from build123d import *

# Parameters (mm, degrees)
F0_W      = 16.51
F0_H      = 21.59
F1_DEPTH  = 3.048
F2_W      = 1.7145
F2_H      = 12.7
F3_DEPTH  = 25.4
F4_W      = 1.5875
F4_H      = 12.7
F5_DEPTH  = 25.4
F7_DEPTH  = 25.4
F8_R      = 1.52399
F9_R      = 1.524
F10_DEPTH = 2.286
F11_R     = 1.524
F12_DEPTH = 2.286
F13_R     = 0.635
F14_R     = 0.635


# Not quite as in the source:
# - a fillet or chamfer is up to 0.001 mm smaller than in the source, because OpenCascade refuses the exact size


with BuildPart() as f1:
    # F0 (on Top) → F1 (new body)
    with BuildSketch(Plane.XY):
        with Locations((8.255, 10.795)):
            Rectangle(F0_W, F0_H)
    extrude(amount=F1_DEPTH)

    # F2 (on face) → F3 (cut)
    with BuildSketch(Plane.XY.offset(3.048)):
        with Locations((4.03225, 15.24)):
            Rectangle(F2_W, F2_H)
    extrude(amount=-F3_DEPTH, mode=Mode.SUBTRACT)

    # F4 (on face) → F5 (cut)
    with BuildSketch(Plane.XY.offset(3.048)):
        with Locations((12.54125, 15.24)):
            Rectangle(F4_W, F4_H)
    extrude(amount=-F5_DEPTH, mode=Mode.SUBTRACT)

    # F6 (on face) → F7 (cut)
    with BuildSketch(Plane(origin=(0, 0, 0), x_dir=(0, -1, 0), z_dir=(-1, 0, 0))):
        Polygon((0, 0), (0, 3.048), (-3.175, 0), align=None)
    extrude(amount=-F7_DEPTH, mode=Mode.SUBTRACT)

    # F8 (radius 1.524 in the source; OpenCascade refuses exactly that, so slightly less here)
    f8_edges = [f1.edges().sort_by_distance(p)[0] for p in [
        (1.5875, 21.59, 3.048),
        (1.5875, 21.59, 0),
        (8.3185, 21.59, 3.048),
        (8.3185, 21.59, 0),
        (14.9225, 21.59, 3.048),
        (14.9225, 21.59, 0),
    ]]
    fillet(f8_edges, radius=F8_R)

    # F9 (on face) → F10 (join)
    with BuildSketch(Plane(origin=(0, 0, 0), x_dir=(0, -1, 0), z_dir=(-1, 0, 0))):
        with Locations((-20.066, 1.524)):
            Circle(F9_R)
    extrude(amount=F10_DEPTH)

    # F11 (on face) → F12 (join)
    with BuildSketch(Plane.YZ.offset(16.51)):
        with Locations((20.066, 1.524)):
            Circle(F11_R)
    extrude(amount=F12_DEPTH)

    # F13
    f13_edges = [f1.edges().sort_by_distance(p)[0] for p in [
        (18.796, 18.542, 1.524),
        (-2.286, 21.59, 1.524),
    ]]
    fillet(f13_edges, radius=F13_R)

    # F14
    f14_edges = [f1.edges().sort_by_distance(p)[0] for p in [
        (11.7475, 8.89, 1.524),
        (13.335, 8.89, 1.524),
        (3.175, 8.89, 1.524),
        (4.8895, 8.89, 1.524),
    ]]
    fillet(f14_edges, radius=F14_R)


solid = f1.part
For this review, take the finished solid that the model builds, in its own axes (mm). A direction names the side the tool comes from. Give positions to 0.01 mm unless a question says otherwise; leave off trailing zeros. Loops run counter-clockwise (first coordinate to the right, second up) from the corner with the lowest first, then second, coordinate; pieces in that order, holes last.
Item 1: Draft analysis for pull direction X (two halves, no side actions). For faces 1 (the flat face through (0, 10, 2)), 2 (the flat face through (4.89, 15, 2)), 3 (the flat face through (8, 12, 0)), state which applies: +X half, -X half, draft (parallel to the pull), parting line (faces both ways), or undercut.
Item 2: Tool access review of faces 4 (the cylindrical face through (17.324, 18.543, 1.591)), 5 (the cylindrical face through (-0.81, 18.66, 0.94)), 6 (the flat face through (11.748, 15, 2)): name each direction out of +Z, -Z, +X, -X, +Y, -Y from which nothing blocks a thin tool from reaching the whole face with its end or side.
Item 3: Take a section at C-C, the plane y = 8. State the section outline as (x, z) points, and give its area (3 significant figures).
Item 4: Take a section at A-A, the plane y = 15. State the section outline as (x, z) points (1 decimal), and give its area (3 significant figures).
Item 5: For line 1 along X through (y, z) = (15.25, 1.45) (1 decimal); line 2 along X through (y, z) = (19.5, 0.8) (1 decimal); line 3 along X through (y, z) = (5.25, 2.25), list the stretches that pass through material, from the lowest coordinate up.
Item 6: Take a section at D-D, the plane x = 3.5. State the section outline as (y, z) points (3 decimals), and give its area (3 significant figures).
Item 7: Insertion check: pin 1 (1.5 mm diameter, centred on y = 13, z = 2, fed in from +X); pin 2 (1.5 mm diameter, centred on x = 1, z = 2, fed in from -Y). Each pin has a flat end and moves straight along its axis. Give the tip position at first contact, or say it passes through.
Calculated:
1. face 1: -X half
1. face 2: undercut
1. face 3: draft
2. face 4: +X
2. face 5: -X
2. face 6: +Z, -Z, +Y
3. outline: (0, 0) - (16.51, 0) - (16.51, 3.05) - (0, 3.05) - close
3. area: 50.3 mm2
4. outline: (0, 0) - (3.2, 0) - (3.2, 3) - (0, 3) - close; (4.9, 0) - (11.7, 0) - (11.7, 3) - (4.9, 3) - close; (13.3, 0) - (16.5, 0) - (16.5, 3) - (13.3, 3) - close
4. area: 40.3 mm2
5. line 1: x = 0 to 3.2, 4.9 to 11.7, 13.3 to 16.5
5. line 2: x = -2.3 to 3.2, 4.9 to 11.7, 13.3 to 18.8
5. line 3: x = 0 to 16.51
6. outline: (0, 3.048) - (3.175, 0) - (8.971, 0) - (8.971, 3.048) - close
6. area: 22.5 mm2
7. pin 1: stops at x = 16.51
7. pin 2: stops at y = 0.31
